```python
from build123d import *

# Parameters (mm, degrees)
F3_DEPTH = 31.75
F5_DEPTH = 5.55725
F6_R     = 5.08


with BuildPart() as f3:
    # F1 (on Front) → F3 (new body)
    with BuildSketch(Plane.XZ):
        Polygon((609.6, 0), (609.6, 5.55625), (520.7, 4.977474), (520.7, 0), align=None)
    extrude(amount=F3_DEPTH)

    # F4 (on face) → F5 (cut, through all)
    with BuildSketch(Plane(origin=(0, 0, 0), x_dir=(1, 0, 0), z_dir=(0, 0, -1))):
        with BuildLine():
            Line((600.075, 25.4), (530.225, 25.4))
            ThreePointArc((530.225, 25.4), (527.979936, 24.470064), (527.05, 22.225))
            Line((527.05, 22.225), (527.05, 9.525))
            ThreePointArc((527.05, 9.525), (527.979936, 7.279936), (530.225, 6.35))
            Line((530.225, 6.35), (600.075, 6.35))
            ThreePointArc((600.075, 6.35), (602.320064, 7.279936), (603.25, 9.525))
            Line((603.25, 9.525), (603.25, 22.225))
            ThreePointArc((603.25, 22.225), (602.320064, 24.470064), (600.075, 25.4))
        make_face()
    extrude(amount=-F5_DEPTH, mode=Mode.SUBTRACT)

    # F6
    f6_edges = [f3.edges().sort_by_distance(p)[0] for p in [
        (520.7, -31.75, 2.488737),
        (520.7, 0, 2.488737),
        (609.6, -31.75, 2.778125),
        (609.6, 0, 2.778125),
    ]]
    fillet(f6_edges, radius=F6_R)


solid = f3.part
```
Check sheet for the modelled part. Datum: model origin and axes. Units: mm. A direction names the side the tool comes from. Round coordinates to 2 decimals unless told otherwise and drop trailing zeros. Order: outer loops, then holes, each group sorted by start corner. A loop starts at its lowest first (then second) coordinate and runs counter-clockwise, first axis right, second up.
1) Mould release check, pull along X, two halves, no side actions. Record for faces 3 (the flat face through (566, -25.4, 3)), 4 (the cylindrical face through (522.228, -30.301, 2.47)), 5 (the flat face through (565, 0, 3)): +X half, -X half, draft (parallel to the pull), parting line (faces both ways), or undercut.
2) Section check A-A (y = -14). Record the boundary of the cut face in (x, z), and give its area (3 significant figures).
3) Tool access check on faces 1 (the flat face through (565, -6.35, 3)), 2 (the cylindrical face through (608.151, -1.528, 2.817)). Record the directions out of +Z, -Z, +X, -X, +Y, -Y that give a thin tool (end or side, any length) a straight path to the whole face; none if there is none.
4) Section check C-C (x = 543). Record the boundary of the cut face in (y, z), and give its area (3 significant figures).
5) Scan lines: line 1 (Y direction, x = 598, z = 4.2); line 2 (X direction, y = -15, z = 3.6); line 3 (X direction, y = -23, z = 4.35). Record each from-to range of solid material in increasing order.
6) Section check B-B (z = 3.45). Record the boundary of the cut face in (x, y) (3 decimals), and give its area (3 significant figures).
Result:
1. face 3: undercut
1. face 4: -X half
1. face 5: draft
2. outline: (520.7, 0) - (527.05, 0) - (527.05, 5.02) - (520.7, 4.98) - close; (603.25, 0) - (609.6, 0) - (609.6, 5.56) - (603.25, 5.51) - close
2. area: 66.9 mm2
3. face 1: +Z, -Z
3. face 2: +Z, -Z, +X, +Y
4. outline: (-31.75, 0) - (-25.4, 0) - (-25.4, 5.12) - (-31.75, 5.12) - close; (-6.35, 0) - (0, 0) - (0, 5.12) - (-6.35, 5.12) - close
4. area: 65.1 mm2
5. line 1: y = -31.75 to -25.4, -6.35 to 0
5. line 2: x = 520.7 to 527.05, 603.25 to 609.6
5. line 3: x = 520.7 to 527.15, 603.15 to 609.6
6. outline: (520.7, -26.67) arc R5.08 ccw to (525.78, -31.75) - (604.52, -31.75) arc R5.08 ccw to (609.6, -26.67) - (609.6, -5.08) arc R5.08 ccw to (604.52, 0) - (525.78, 0) arc R5.08 ccw to (520.7, -5.08) - close; hole (527.05, -22.225) arc R3.175 ccw to (530.225, -25.4) - (600.075, -25.4) arc R3.175 ccw to (603.25, -22.225) - (603.25, -9.525) arc R3.175 ccw to (600.075, -6.35) - (530.225, -6.35) arc R3.175 ccw to (527.05, -9.525) - close
6. area: 1,360 mm2
